Work out the finished part from the listing and answer in its coordinate system (mm). A direction names the side the tool comes from. Round coordinates to 2 decimals unless told otherwise and drop trailing zeros. Write each loop counter-clockwise with the first axis right and the second up, starting at its lowest first coordinate (ties: lowest second). Pieces come first, ordered by that corner, then holes. Notation, with made-up numbers: (0, -17.75) - (22, -17.75) arc R24 ccw to (22, 1.25) - close; hole circle Ø2 at (-37, -8.75). An arc over 180 degrees is marked (long way). Write item = value, one per line. Start each with the question number.
from build123d import *

# Parameters (mm, degrees)
F0_W     = 122.23322317
F0_H     = 26.7385169864
F1_DEPTH = 45
F2_DEPTH = 40
F3_DEPTH = 40


with BuildPart() as f1:
    # F0 (on Front) → F1 (new body, symmetric)
    with BuildSketch(Plane.XZ):
        with BuildLine():
            Line((-57.0032522082, 75.0096067786), (-64.3862187862, 75.0096067786))
            Line((-64.3862187862, 75.0096067786), (-64.3862187862, -74.3724256754))
            Line((-64.3862187862, -74.3724256754), (0, -74.3724256754))
            Line((0, -74.3724256754), (64.3862187862, -74.3724256754))
            Line((64.3862187862, -74.3724256754), (64.3862187862, 52.1305650473))
            Line((64.3862187862, 52.1305650473), (57.0032522082, 52.1305650473))
            Line((57.0032522082, 52.1305650473), (57.0032522082, 15.2034306045))
            ThreePointArc((57.0032522082, 15.2034306045), (41.1532258631, -24.2843129669), (2.40046245, -41.8549861284))
            ThreePointArc((2.40046245, -41.8549861284), (-0.213800426, -43.1045012545), (-2.8236144574, -41.8457204329))
            ThreePointArc((-2.8236144574, -41.8457204329), (-39.6712510694, -25.9900753758), (-57.0032522082, 10.1865958446))
            Line((-57.0032522082, 10.1865958446), (-57.0032522082, 75.0096067786))
        make_face()
        with Locations((0.1888852566, -56.8894036114)):
            Rectangle(F0_W, F0_H, mode=Mode.SUBTRACT)
        with BuildLine():
            Line((57.0032522082, 75.0096067786), (-57.0032522082, 75.0096067786))
            Line((-57.0032522082, 75.0096067786), (-57.0032522082, 10.1865958446))
            ThreePointArc((-57.0032522082, 10.1865958446), (-39.6712510694, -25.9900753758), (-2.8236144574, -41.8457204329))
            ThreePointArc((-2.8236144574, -41.8457204329), (-0.2116819988, -41.9101142032), (2.40046245, -41.8549861284))
            ThreePointArc((2.40046245, -41.8549861284), (41.1532258631, -24.2843129669), (57.0032522082, 15.2034306045))
            Line((57.0032522082, 15.2034306045), (57.0032522082, 52.1305650473))
            Line((57.0032522082, 52.1305650473), (57.0032522082, 75.0096067786))
        make_face()
        with Locations((0.1888852566, -56.8894036114)):
            Rectangle(F0_W, F0_H)
        with BuildLine():
            ThreePointArc((2.40046245, -41.8549861284), (-0.2116819988, -41.9101142032), (-2.8236144574, -41.8457204329))
            ThreePointArc((-2.8236144574, -41.8457204329), (-0.213800426, -43.1045012545), (2.40046245, -41.8549861284))
        make_face()
    extrude(amount=F1_DEPTH, both=True)

    # F0 (on Front) → F2 (cut, symmetric)
    with BuildSketch(Plane.XZ):
        with BuildLine():
            Line((57.0032522082, 75.0096067786), (-57.0032522082, 75.0096067786))
            Line((-57.0032522082, 75.0096067786), (-57.0032522082, 10.1865958446))
            ThreePointArc((-57.0032522082, 10.1865958446), (-39.6712510694, -25.9900753758), (-2.8236144574, -41.8457204329))
            ThreePointArc((-2.8236144574, -41.8457204329), (-0.2116819988, -41.9101142032), (2.40046245, -41.8549861284))
            ThreePointArc((2.40046245, -41.8549861284), (41.1532258631, -24.2843129669), (57.0032522082, 15.2034306045))
            Line((57.0032522082, 15.2034306045), (57.0032522082, 52.1305650473))
            Line((57.0032522082, 52.1305650473), (57.0032522082, 75.0096067786))
        make_face()
        with BuildLine():
            ThreePointArc((2.40046245, -41.8549861284), (-0.2116819988, -41.9101142032), (-2.8236144574, -41.8457204329))
            ThreePointArc((-2.8236144574, -41.8457204329), (-0.213800426, -43.1045012545), (2.40046245, -41.8549861284))
        make_face()
    extrude(amount=F2_DEPTH, both=True, mode=Mode.SUBTRACT)

    # F0 (on Front) → F3 (cut, symmetric)
    with BuildSketch(Plane.XZ):
        with Locations((0.1888852566, -56.8894036114)):
            Rectangle(F0_W, F0_H)
    extrude(amount=F3_DEPTH, both=True, mode=Mode.SUBTRACT)


solid = f1.part
1. Find section D-D on x = 7. Give the vertices of the cut face in (y, z), plus the area to 3 significant figures.
2. Each of these flat-tipped pins is pushed along its axis until it touches: pin 1 (5.5 mm diameter, centred on y = 43.5, z = 63.5, fed in from +X); pin 2 (8 mm diameter, centred on x = 18.5, y = 22.5, fed in from +Z); pin 3 (8 mm diameter, centred on x = -21, y = -0.5, fed in from +Z). Where does it stop, or does it pass through?
3. Consider line 1 (Y direction, x = -41, z = 52.5); line 2 (X direction, y = -2, z = -49.5); line 3 (X direction, y = -22.5, z = 28.5). Determine where each line is inside the solid, lowest interval first.
4. Which of the six approach directions +Z, -Z, +X, -X, +Y, -Y give full straight-line access (tool end or side, diameter ignored) to faces 5 (the face through (57.003, -43, 63)), 6 (the face through (57.003, -1, 33)), 7 (the face through (-1, 40, -57)), 8 (the face through (-1, 45, 1))?
5. Find section C-C on z = -57. Give the vertices of the cut face in (x, y).
6. For a pull along Z with two mould halves and no side action, classify faces 1 (the face through (-1, -40, 17)), 2 (the face through (-1, -1, -43.52)), 3 (the face through (61, -1, 52.131)), 4 (the face through (-1, -1, -70.259)) as released by +Z, released by -Z, zero draft, split by the parting line, or undercut.
7. Find section B-B on y = 11. Give the vertices of the cut face in (x, z), plus the area to 3 significant figures.
8. Find section A-A on z = 62. Give the vertices of the cut face in (x, y).
Answer key:
q1.outline = (-45, -74.37) - (45, -74.37) - (45, 75.01) - (40, 75.01) - (40, -41.47) - (-40, -41.47) - (-40, 75.01) - (-45, 75.01) - close; hole (-40, -70.26) - (40, -70.26) - (40, -43.52) - (-40, -43.52) - close
q1.area = 1,990 mm²
q2.pin_1 = 57
q2.pin_2 = -37.24
q2.pin_3 = -36.2
q3.line_1 = -45 to -40, 40 to 45
q3.line_2 = -64.39 to -60.93, 61.31 to 64.39
q3.line_3 = -64.39 to -57, 57 to 64.39
q4.face_5 = +Z, +X, +Y, -Y
q4.face_6 = +Z
q4.face_7 = none
q4.face_8 = +Z, -Z, +X, -X, +Y
q5.outline = (-64.39, -45) - (64.39, -45) - (64.39, 45) - (-64.39, 45) - close; hole (-60.93, -40) - (61.31, -40) - (61.31, 40) - (-60.93, 40) - close
q6.face_1 = zero draft
q6.face_2 = undercut
q6.face_3 = released by +Z
q6.face_4 = undercut
q7.outline = (-64.39, -74.37) - (64.39, -74.37) - (64.39, 52.13) - (57, 52.13) - (57, 15.2) arc R57.11 cw to (2.4, -41.85) arc R3.35 cw to (-2.82, -41.85) arc R57.11 cw to (-57, 10.19) - (-57, 75.01) - (-64.39, 75.01) - close; hole (-60.93, -70.26) - (61.31, -70.26) - (61.31, -43.52) - (-60.93, -43.52) - close
q7.area = 3,850 mm²
q8.outline = (-64.39, -45) - (57, -45) - (57, -40) - (-57, -40) - (-57, 40) - (57, 40) - (57, 45) - (-64.39, 45) - close
